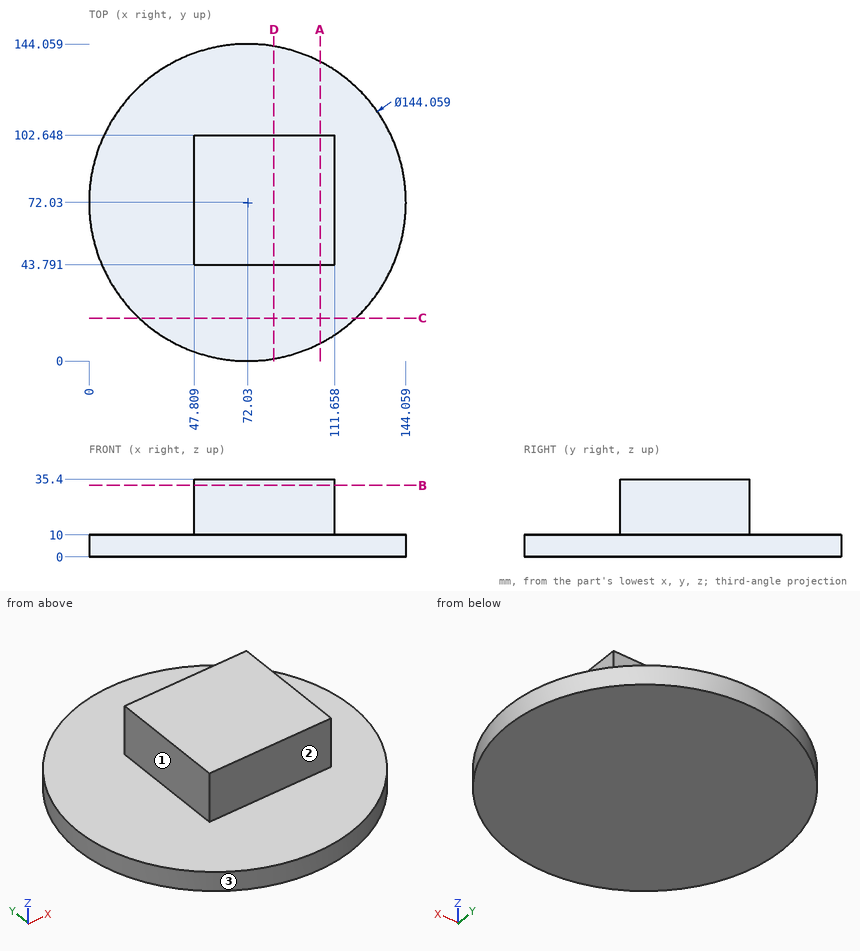
Input: dimensioned drawing with shaded views. Units: mm. Origin: part minimum x, y, z. A direction names the side the tool comes from. Give positions to 0.01 mm unless a question says otherwise; leave off trailing zeros. Write each loop counter-clockwise with the first axis right and the second up, starting at its lowest first coordinate (ties: lowest second). Pieces come first, ordered by that corner, then holes. Notation, with made-up numbers: (-16.75, -14) - (7.25, -14) arc R11 ccw to (7.25, 7) - close; hole circle Ø8 at (3, -36.75). An arc over 180 degrees is marked (long way). One line per item, written item: value. Start each with the question number.
Q1. First-contact query: pin 1 Ø2 at (y, z) = (57, 28) entering from +X; pin 2 Ø4 at (y, z) = (79.5, 6.5) entering from +X; pin 3 Ø5 at (x, z) = (63, 18.5) entering from +Y. Flat tips, straight axial feed; report the tip coordinate or a pass-through.
Q2. Section query C-C, the plane y = 19.5. Return the cut outline in (x, z) (1 decimal), then the cut area to 3 significant figures.
Q3. Set-up query: the marked faces 1, 2 and 3. Return all of +Z, -Z, +X, -X, +Y, -Y with unobstructed straight access to the full face (end or side cutting, diameter ignored); none if empty.
Q4. Material intervals for probe 1 along Z at (x, y) = (120.5, 43.5); probe 2 along X at (y, z) = (59, 28.5); probe 3 along Y at (x, z) = (76, 34), sorted ascending. Write a range as from..to.
Q5. Section query D-D, the plane x = 84. Return the cut outline in (y, z), then the cut area to 3 significant figures.
Q6. Section query A-A, the plane x = 105. Return the cut outline in (y, z), then the cut area to 3 significant figures.
Q7. Section query B-B, the plane z = 32.5. Return the cut outline in (x, y), then the cut area to 3 significant figures.
Answer:
1. pin 1: stops at x = 111.66
1. pin 2: stops at x = 143.85
1. pin 3: stops at y = 102.65
2. outline: (22.7, 0) - (121.3, 0) - (121.3, 10) - (22.7, 10) - close
2. area: 986 mm2
3. face 1: +Z, -X, +Y, -Y
3. face 2: +Z, +X, -X, -Y
3. face 3: +Z, -Z
4. probe 1: z = 0..10
4. probe 2: x = 47.81..111.66
4. probe 3: y = 43.79..102.65
5. outline: (1, 0) - (143.06, 0) - (143.06, 10) - (102.65, 10) - (102.65, 35.4) - (43.79, 35.4) - (43.79, 10) - (1, 10) - close
5. area: 2,920 mm2
6. outline: (7.99, 0) - (136.07, 0) - (136.07, 10) - (102.65, 10) - (102.65, 35.4) - (43.79, 35.4) - (43.79, 10) - (7.99, 10) - close
6. area: 2,780 mm2
7. outline: (47.81, 43.79) - (111.66, 43.79) - (111.66, 102.65) - (47.81, 102.65) - close
7. area: 3,760 mm2
